from build123d import *

# Parameters (mm, degrees)
SKETCH_1_R          = 14
SKETCH_1_R_2        = 1.5
EXTRUDE_1_DEPTH     = 2
CUT_EXTRUDE_1_DEPTH = 20.899748742


with BuildPart() as part:
    # 草图1 → 凸台-拉伸1 (new body)
    with BuildSketch(Plane.XY):
        Circle(SKETCH_1_R)
        with Locations((-7.071067812, 7.071067812)):
            Circle(SKETCH_1_R_2, mode=Mode.SUBTRACT)
        with Locations((7.071067812, 7.071067812)):
            Circle(SKETCH_1_R_2, mode=Mode.SUBTRACT)
        with Locations((-7.071067812, -7.071067812)):
            Circle(SKETCH_1_R_2, mode=Mode.SUBTRACT)
        with Locations((7.071067812, -7.071067812)):
            Circle(SKETCH_1_R_2, mode=Mode.SUBTRACT)
    extrude(amount=EXTRUDE_1_DEPTH)

    # 草图2 → 切除-拉伸1 (cut, through all)
    with BuildSketch(Plane(origin=(0, 0, 0), x_dir=(-1, 0, 0), z_dir=(0, 0, -1))):
        with BuildLine():
            Line((-2.856571371, 2.8), (2.856571371, 2.8))
            ThreePointArc((2.856571371, 2.8), (4, 0), (2.856571371, -2.8))
            Line((2.856571371, -2.8), (-2.856571371, -2.8))
            ThreePointArc((-2.856571371, -2.8), (-4, 0), (-2.856571371, 2.8))
        make_face()
    extrude(amount=-CUT_EXTRUDE_1_DEPTH, mode=Mode.SUBTRACT)


solid = part.part
The model under review builds one solid part; all positions refer to its coordinate system, in mm. A direction names the side the tool comes from. Give positions to 0.01 mm unless a question says otherwise; leave off trailing zeros. Write each loop counter-clockwise with the first axis right and the second up, starting at its lowest first coordinate (ties: lowest second). Pieces come first, ordered by that corner, then holes.
1. Add section D-D, the plane y = 6.75. Write out the cut boundary in (x, z), plus the area to 3 significant figures.
2. Add section B-B, the plane y = 0. Write out the cut boundary in (x, z).
3. Draft analysis for pull direction Y (two halves, no side actions). For faces 3 (the flat face through (0, -3, 2)), 4 (the cylindrical face through (-5.685, 6.497, 0.986)), 5 (the cylindrical face through (12.932, -5.362, 0.986)), 6 (the cylindrical face through (-4, 0, 1)), state which applies: +Y half, -Y half, draft (parallel to the pull), parting line (faces both ways), or undercut.
4. Wall thickness on L1, parallel to X at y = 8.25, z = 1.4; L2, parallel to X at y = -6.25, z = 1.1; L3, parallel to Y at x = 6.5, z = 0.15: over which ranges is each line inside the solid? List them lowest first.
5. For P1, Ø1, axis at x = 0.5, z = 0.5, coming from the +Y side, flat-tipped, find the tip position at first contact; note if it passes through.
6. Tool access review of faces 1 (the flat face through (0, -3, 0)), 2 (the flat face through (0, 2.8, 1)): name each direction out of +Z, -Z, +X, -X, +Y, -Y from which nothing blocks a thin tool from reaching the whole face with its end or side.
7. Add section C-C, the plane z = 1.65. Write out the cut boundary in (x, y), plus the area to 3 significant figures.
8. Add section A-A, the plane x = 0. Write out the cut boundary in (y, z).
Worked answers:
1. outline: (-12.27, 0) - (-8.54, 0) - (-8.54, 2) - (-12.27, 2) - close; (-5.61, 0) - (5.61, 0) - (5.61, 2) - (-5.61, 2) - close; (8.54, 0) - (12.27, 0) - (12.27, 2) - (8.54, 2) - close
1. area: 37.3 mm2
2. outline: (-14, 0) - (-4, 0) - (-4, 2) - (-14, 2) - close; (4, 0) - (14, 0) - (14, 2) - (4, 2) - close
3. face 3: draft
3. face 4: undercut
3. face 5: parting line
3. face 6: undercut
4. L1: x = -11.31 to -8, -6.14 to 6.14, 8 to 11.31
4. L2: x = -12.53 to -8.33, -5.82 to 5.82, 8.33 to 12.53
4. L3: y = -12.4 to -8.46, -5.68 to 5.68, 8.46 to 12.4
5. P1: stops at y = 14
6. face 1: -Z, +X, -X, +Y, -Y
6. face 2: +Z, -Z
7. outline: circle Ø28 at (0, 0); hole circle Ø3 at (-7.07, -7.07); hole circle Ø3 at (-7.07, 7.07); hole (-2.86, -2.8) - (2.86, -2.8) arc R4 ccw to (2.86, 2.8) - (-2.86, 2.8) arc R4 ccw to start; hole circle Ø3 at (7.07, -7.07); hole circle Ø3 at (7.07, 7.07)
7. area: 547 mm2
8. outline: (-14, 0) - (-2.8, 0) - (-2.8, 2) - (-14, 2) - close; (2.8, 0) - (14, 0) - (14, 2) - (2.8, 2) - close
